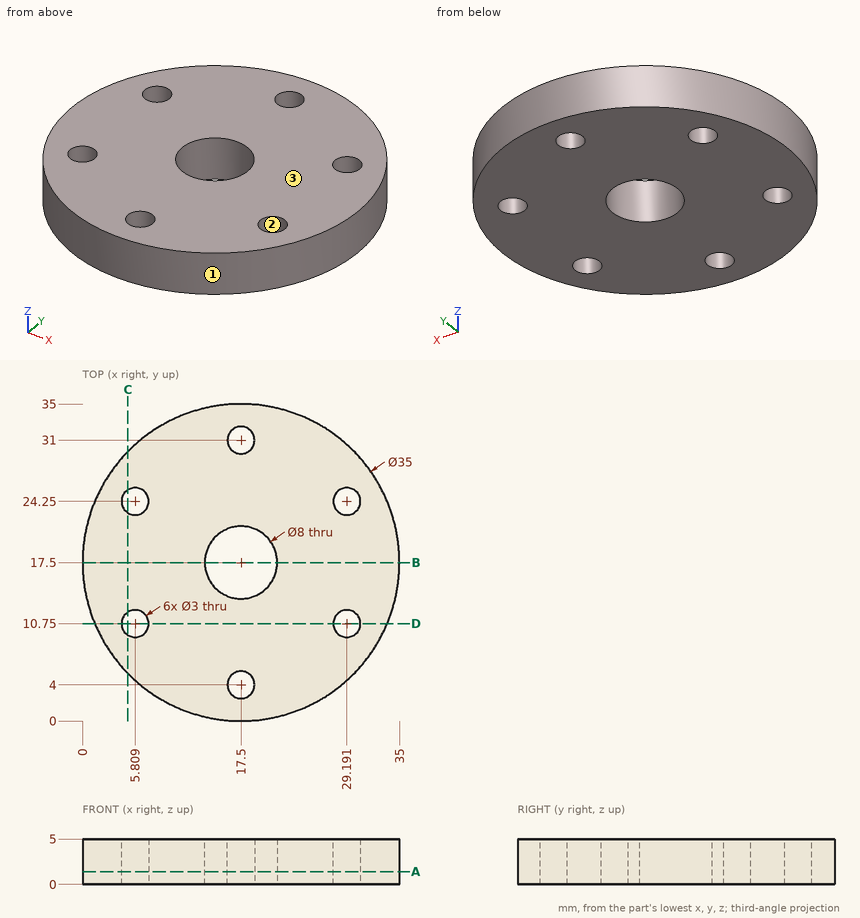
Part print with two shaded views. Sizes in mm from the minimum x, y, z corner. Round coordinates to 2 decimals unless told otherwise and drop trailing zeros. Loops run counter-clockwise (first coordinate to the right, second up) from the corner with the lowest first, then second, coordinate; pieces in that order, holes last. Notation, with made-up numbers: M 39,45.25 L 81,45.25 A31 cw 81,69.25 Z; hole C 89.25,-10.5 d3. An arc over 180 degrees is marked long. Put each result on its own line as item: value. Start each with the question number.
Item 1: Cut at B-B (y = 17.5). List the corners of the cut face in (x, z), then the cut area to 3 significant figures.
Item 2: Mould opens along X. For the marked faces 1, 2 and 3 say: released by +X, released by -X, zero draft, split by the parting line, or undercut.
Item 3: Cut at C-C (x = 5). List the corners of the cut face in (y, z).
Item 4: Drill centre lines: line 1 along Y through (x, z) = (17.5, 3.15); line 2 along X through (y, z) = (23.5, 1.65); line 3 along X through (y, z) = (23, 4.45) (1 decimal). Where is each one in solid material? Low to high.
Item 5: Drop flat-ended pins along their axis: P1, Ø1.5, axis at y = 15, z = 0.5, coming from the +X side; P2, Ø1.5, axis at x = 19.5, z = 2.5, coming from the -Y side (1 decimal); P3, Ø1, axis at x = 25.5, z = 3.5, coming from the -Y side. Give the stop position or say it passes through.
Item 6: Cut at D-D (y = 10.75). List the corners of the cut face in (x, z).
Item 7: Cut at A-A (z = 1.4). List the corners of the cut face in (x, y).
Answer block:
1. outline: M 0,0 L 13.5,0 L 13.5,5 L 0,5 Z; M 21.5,0 L 35,0 L 35,5 L 21.5,5 Z
1. area: 135 mm2
2. face 1: split by the parting line
2. face 2: undercut
2. face 3: zero draft
3. outline: M 5.25,0 L 9.49,0 L 9.49,5 L 5.25,5 Z; M 12.01,0 L 22.99,0 L 22.99,5 L 12.01,5 Z; M 25.51,0 L 29.75,0 L 29.75,5 L 25.51,5 Z
4. line 1: 0 to 2.5, 5.5 to 13.5, 21.5 to 29.5, 32.5 to 35
4. line 2: 1.06 to 4.51, 7.11 to 27.89, 30.49 to 33.94
4. line 3: 0.9 to 5, 6.6 to 28.4, 30 to 34.1
5. P1: x = 34.91
5. P2: y = 0
5. P3: y = 1.69
6. outline: M 1.35,0 L 4.31,0 L 4.31,5 L 1.35,5 Z; M 7.31,0 L 27.69,0 L 27.69,5 L 7.31,5 Z; M 30.69,0 L 33.65,0 L 33.65,5 L 30.69,5 Z
7. outline: C 17.5,17.5 d35; hole C 5.81,10.75 d3; hole C 5.81,24.25 d3; hole C 17.5,17.5 d8; hole C 17.5,4 d3; hole C 17.5,31 d3; hole C 29.19,10.75 d3; hole C 29.19,24.25 d3
